Part model, mm, in its own coordinate system. A direction names the side the tool comes from. Coordinates: 2 decimals unless noted, no trailing zeros. Write each loop counter-clockwise with the first axis right and the second up, starting at its lowest first coordinate (ties: lowest second). Pieces come first, ordered by that corner, then holes. Notation, with made-up numbers: (-35.5, 32.5) -> (11.5, 32.5) arc R18 cw to (11.5, 52.5) -> close; hole circle Ø4 at (5.5, 54.5). An arc over 180 degrees is marked (long way). Write item = value, one per line. Start each with the question number.
Q1. Probe line 1 (X direction, y = 13.5, z = 13); line 2 (Y direction, x = -30, z = 7.25) (3 decimals); line 3 (Y direction, x = 0, z = 14). List the from-to ranges inside material, lowest first.
Q2. Pull direction Y, two halves, no side cores. Call faces 5 (the flat face through (-23, 9.575, 15)), 6 (the cylindrical face through (-34.621, 18.072, 15.38)), 7 (the cylindrical face through (-25.046, 16.984, 11.232)): released by +Y, released by -Y, zero draft, split by the parting line, or undercut.
Q3. Band-saw the part on B-B, the plane z = 13.75. Give the number of separate pieces and of enclosed holes in the cut face, plus the area to 3 significant figures.
Q4. Tool access for faces 1 (the flat face through (9, 8.235, 15)), 2 (the flat face through (-34.072, 12, 15)), 3 (the flat face through (34.072, 12, 15)), 4 (the flat face through (24, 16.5, 15)): list every direction of +Z, -Z, +X, -X, +Y, -Y with a clear straight run to the whole face (end or side of a thin tool).
Q5. Band-saw the part on A-A, the plane x = 21. List the corners of the cut face in (y, z).
Q6. Pin check, flat tips, straight feed: P1, Ø0.7, axis at y = 10, z = 18, coming from the +X side; P2, Ø2, axis at y = 10.5, z = 16.5, coming from the +X side; P3, Ø1.5, axis at x = 19.5, y = 12.5, coming from the -Z side. Stop position of each tip, or through.
from build123d import *

# Parameters (mm, degrees)
F2_DEPTH  = 18.5
F3_R      = 1.55
F4_DEPTH  = 3.075
F5_W      = 6
F5_H      = 0.5
F6_DEPTH  = 0.2
F5_W_2    = 4
F5_H_2    = 2.25
F7_DEPTH  = 0.6
F8_W      = 4
F8_H      = 0.5
F9_DEPTH  = 0.9
F8_H_2    = 0.47
F10_DEPTH = 0.2
F11_W     = 4
F11_H     = 0.5
F12_DEPTH = 0.9
F11_H_2   = 0.47
F13_DEPTH = 0.2
F14_W     = 4
F14_H     = 0.5
F15_DEPTH = 0.7
F16_W     = 8
F16_H     = 7
F17_DEPTH = 1
F17_TAPER = 45
F18_W     = 8
F18_H     = 7
F19_DEPTH = 1
F19_TAPER = 45
F22_ANGLE = 90


with BuildPart() as f2:
    # F1 (on Front) → F2 (new body)
    with BuildSketch(Plane.XZ):
        with BuildLine():
            Line((-33.5725, -6), (33.5725, -6))
            ThreePointArc((33.5725, -6), (34.6331601718, -5.5606601718), (35.0725, -4.5))
            Line((35.0725, -4.5), (35.0725, 4.5))
            ThreePointArc((35.0725, 4.5), (34.6331601718, 5.5606601718), (33.5725, 6))
            Line((33.5725, 6), (-33.5725, 6))
            ThreePointArc((-33.5725, 6), (-34.6331601718, 5.5606601718), (-35.0725, 4.5))
            Line((-35.0725, 4.5), (-35.0725, -4.5))
            ThreePointArc((-35.0725, -4.5), (-34.6331601718, -5.5606601718), (-33.5725, -6))
        make_face()
        with BuildLine():
            ThreePointArc((-14.9225, -0.925), (-15.5082864376, -2.3392135624), (-16.9225, -2.925))
            Line((-16.9225, -2.925), (-30.0725, -2.925))
            ThreePointArc((-30.0725, -2.925), (-31.4867135624, -2.3392135624), (-32.0725, -0.925))
            Line((-32.0725, -0.925), (-32.0725, 0.925))
            ThreePointArc((-32.0725, 0.925), (-31.4867135624, 2.3392135624), (-30.0725, 2.925))
            Line((-30.0725, 2.925), (-16.9225, 2.925))
            ThreePointArc((-16.9225, 2.925), (-15.5082864376, 2.3392135624), (-14.9225, 0.925))
            Line((-14.9225, 0.925), (-14.9225, -0.925))
        make_face(mode=Mode.SUBTRACT)
        with BuildLine():
            Line((-9.6675, 4.265), (-1.0875, 4.265))
            ThreePointArc((-1.0875, 4.265), (-0.0268398282, 3.8256601718), (0.4125, 2.765))
            Line((0.4125, 2.765), (0.4125, -2.765))
            ThreePointArc((0.4125, -2.765), (-0.0268398282, -3.8256601718), (-1.0875, -4.265))
            Line((-1.0875, -4.265), (-9.6675, -4.265))
            ThreePointArc((-9.6675, -4.265), (-10.7281601718, -3.8256601718), (-11.1675, -2.765))
            Line((-11.1675, -2.765), (-11.1675, 2.765))
            ThreePointArc((-11.1675, 2.765), (-10.7281601718, 3.8256601718), (-9.6675, 4.265))
        make_face(mode=Mode.SUBTRACT)
        with BuildLine():
            Line((4.3325, 4.265), (12.9125, 4.265))
            ThreePointArc((12.9125, 4.265), (13.9731601718, 3.8256601718), (14.4125, 2.765))
            Line((14.4125, 2.765), (14.4125, -2.765))
            ThreePointArc((14.4125, -2.765), (13.9731601718, -3.8256601718), (12.9125, -4.265))
            Line((12.9125, -4.265), (4.3325, -4.265))
            ThreePointArc((4.3325, -4.265), (3.2718398282, -3.8256601718), (2.8325, -2.765))
            Line((2.8325, -2.765), (2.8325, 2.765))
            ThreePointArc((2.8325, 2.765), (3.2718398282, 3.8256601718), (4.3325, 4.265))
        make_face(mode=Mode.SUBTRACT)
        with BuildLine():
            ThreePointArc((32.0725, -3.8), (32.0139213562, -3.9414213562), (31.8725, -4))
            Line((31.8725, -4), (17.0725, -4))
            ThreePointArc((17.0725, -4), (16.9310786438, -3.9414213562), (16.8725, -3.8))
            Line((16.8725, -3.8), (16.8725, 3.8))
            ThreePointArc((16.8725, 3.8), (16.9310786438, 3.9414213562), (17.0725, 4))
            Line((17.0725, 4), (31.8725, 4))
            ThreePointArc((31.8725, 4), (32.0139213562, 3.9414213562), (32.0725, 3.8))
            Line((32.0725, 3.8), (32.0725, -3.8))
        make_face(mode=Mode.SUBTRACT)
    extrude(amount=-F2_DEPTH)

    # F3 (on face) → F4 (cut, through all)
    with BuildSketch(Plane.XY.offset(6)):
        with Locations((-23.4975, 13.2)):
            Circle(F3_R)
    extrude(amount=-F4_DEPTH, mode=Mode.SUBTRACT)

    # F5 (on face) → F6 (join)
    with BuildSketch(Plane.XY.offset(-2.925)):
        with Locations((-23.4975, 18.25)):
            Rectangle(F5_W, F5_H)
    extrude(amount=F6_DEPTH)

    # F5 (on face) → F7 (join)
    with BuildSketch(Plane.XY.offset(-2.925)):
        with Locations((-23.4975, 6.575)):
            Rectangle(F5_W_2, F5_H_2)
    extrude(amount=F7_DEPTH)

    # F8 (on face) → F9 (join)
    with BuildSketch(Plane.XY.offset(-4.265)):
        with Locations((-5.3775, 18.25)):
            Rectangle(F8_W, F8_H)
    extrude(amount=F9_DEPTH)

    # F8 (on face) → F10 (join)
    with BuildSketch(Plane.XY.offset(-4.265)):
        with Locations((-5.3775, 0.235)):
            Rectangle(F8_W, F8_H_2)
    extrude(amount=F10_DEPTH)

    # F11 (on face) → F12 (join)
    with BuildSketch(Plane.XY.offset(-4.265)):
        with Locations((8.6225, 18.25)):
            Rectangle(F11_W, F11_H)
    extrude(amount=F12_DEPTH)

    # F11 (on face) → F13 (join)
    with BuildSketch(Plane.XY.offset(-4.265)):
        with Locations((8.6225, 0.235)):
            Rectangle(F11_W, F11_H_2)
    extrude(amount=F13_DEPTH)

    # F14 (on face) → F15 (join)
    with BuildSketch(Plane.XY.offset(-4)):
        with Locations((24.4725, 18.25)):
            Rectangle(F14_W, F14_H)
    extrude(amount=F15_DEPTH)

    # F16 (on face) → F17 (cut)
    with BuildSketch(Plane.YZ.offset(35.0725)):
        with Locations((9.25, 0)):
            Rectangle(F16_W, F16_H)
    extrude(amount=-F17_DEPTH, taper=F17_TAPER, mode=Mode.SUBTRACT)

    # F18 (on face) → F19 (cut)
    with BuildSketch(Plane(origin=(-35.0725, 0, 0), x_dir=(0, -1, 0), z_dir=(-1, 0, 0))):
        with Locations((-9.25, 0)):
            Rectangle(F18_W, F18_H)
    extrude(amount=-F19_DEPTH, taper=F19_TAPER, mode=Mode.SUBTRACT)


with BuildPart() as f2_1:
    # F22: moved
    add(f2.part.rotate(Axis((0, 18.5, 6), (-1, 0, 0)), F22_ANGLE))


solid = f2_1.part
Ans:
q1.line_1 = -34.07 to -32.07, -14.92 to -11.17, 0.41 to 2.83, 14.41 to 16.87, 32.07 to 34.07
q1.line_2 = 6.5 to 9.575, 15.425 to 18.5
q1.line_3 = 6.5 to 8.7, 16.3 to 18.5
q2.face_5 = undercut
q2.face_6 = released by +Y
q2.face_7 = zero draft
q3.separate_pieces = 1
q3.enclosed_holes = 4
q3.area = 416 mm2
q4.face_1 = none
q4.face_2 = -X
q4.face_3 = +X
q4.face_4 = +Z, -Z
q5.outline = (6.5, 6) -> (8.5, 6) -> (8.5, 24.5) -> (6.5, 24.5) -> close; (16.5, 6) -> (18.5, 6) -> (18.5, 24.5) -> (16.5, 24.5) -> close
q6.P1 = 34.42
q6.P2 = 34.57
q6.P3 = through
